Geometry check sheet. Reference: drawing and pictorial views, mm from the part's lowest x, y, z. Give positions to 0.01 mm unless a question says otherwise; leave off trailing zeros. Order: outer loops, then holes, each group sorted by start corner. A loop starts at its lowest first (then second) coordinate and runs counter-clockwise, first axis right, second up. Notation, with made-up numbers: M 51.5,-27.75 L 89.5,-27.75 A6 ccw 89.5,-22.75 Z; hole C -20.75,-35.5 d7. An arc over 180 degrees is marked long. Answer as CSV lines item,"result".
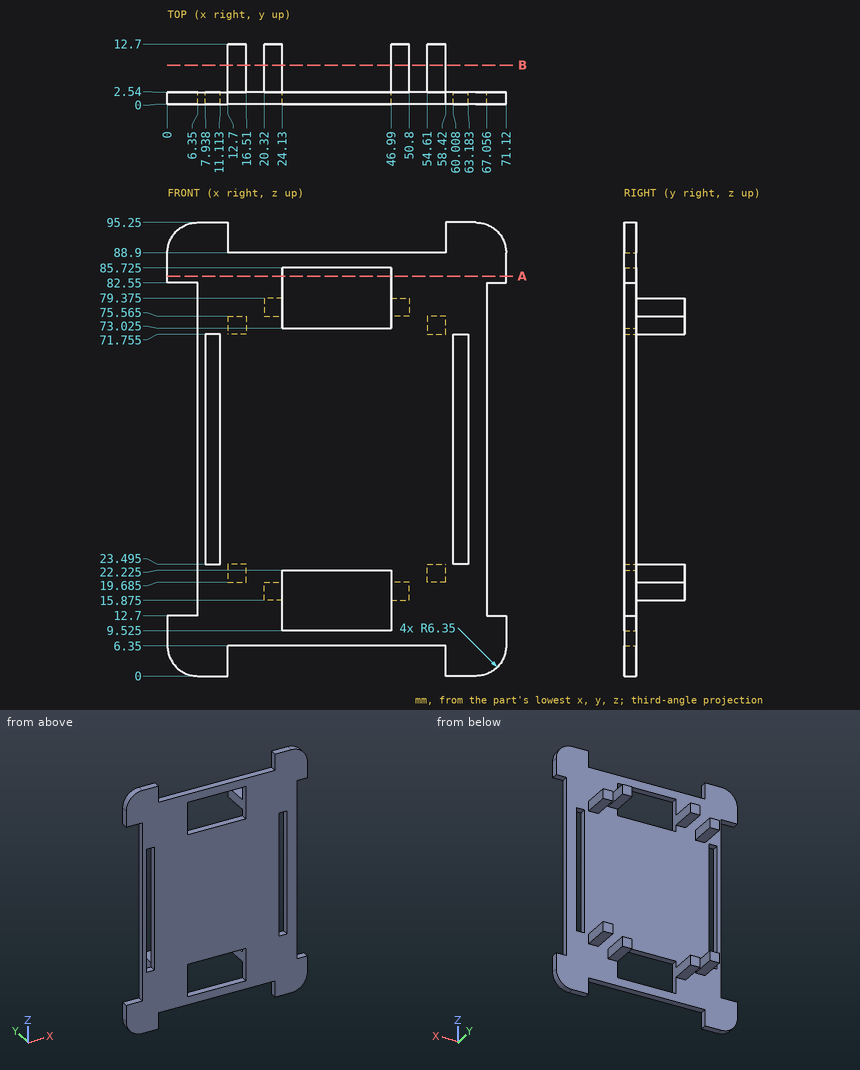
(1) Gauge pin test, flat ends, axial feed: P1, Ø6, axis at y = 6, z = 53, coming from the +X side; P2, Ø4, axis at x = 24, y = 9, coming from the +Z side (1 decimal); P3, Ø3, axis at x = 49.5, y = 6, coming from the -Z side (1 decimal); P4, Ø5, axis at x = 16, y = 6, coming from the -Z side (1 decimal). Record the tip position at first contact, or that the pin passes through.
The answers:
P1,"passes through"
P2,"stops at z = 79.4"
P3,"stops at z = 15.9"
P4,"stops at z = 19.7"
(2) Material ranges on line 1 (Z direction, x = 23, y = 3.75) (1 decimal); line 2 (Y direction, x = 65, z = 51); line 3 (Z direction, x = 17, y = 2), recorded low to high.
The answers:
line 1,"z = 15.9 to 19.7, 75.6 to 79.4"
line 2,"y = 0 to 2.54"
line 3,"z = 6.35 to 88.9"
(3) Section check A-A on z = 84. Enter the section's corners in (x, y).
The answers:
outline,"M 0,0 L 24.13,0 L 24.13,2.54 L 0,2.54 Z; M 46.99,0 L 71.12,0 L 71.12,2.54 L 46.99,2.54 Z"
(4) Section check B-B on y = 8.25. State how many separate pieces and enclosed holes the cut face has, then the cut area to 3 significant figures.
The answers:
separate pieces,"8"
enclosed holes,"0"
area,"116 mm2"
